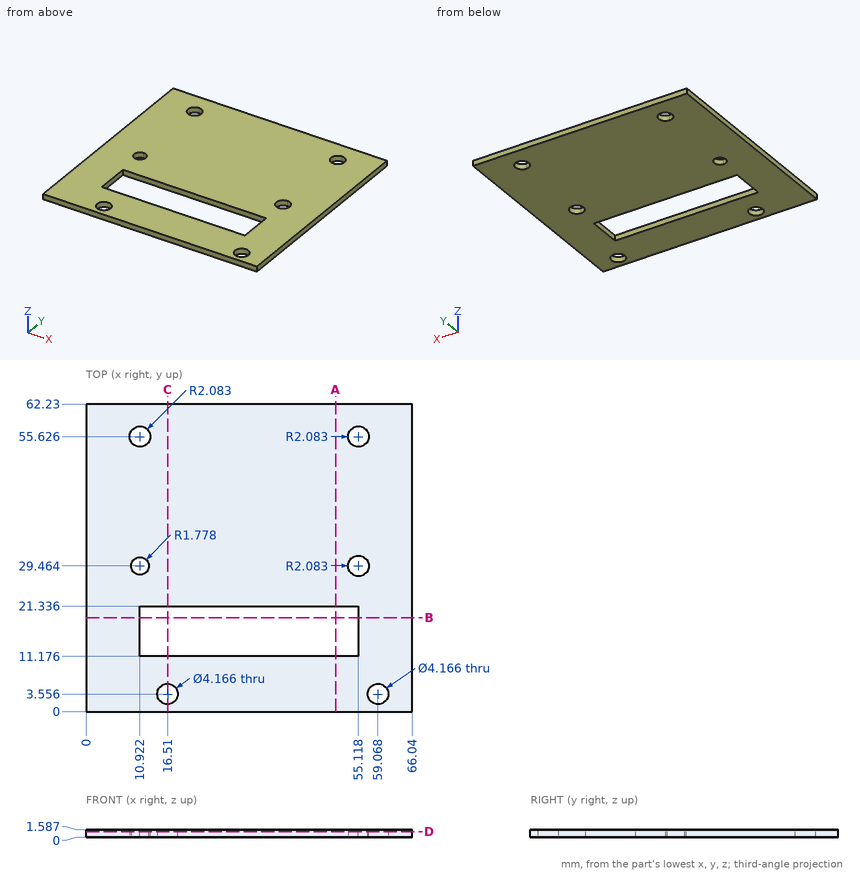
Geometry: see drawing. Coordinates: mm, zero at the bounding-box minimum. Coordinates: 2 decimals unless noted, no trailing zeros. Loops run counter-clockwise (first coordinate to the right, second up) from the corner with the lowest first, then second, coordinate; pieces in that order, holes last. Notation, with made-up numbers: (-12, 77) - (43, 77) arc R20 ccw to (43, 108) - close; hole circle Ø10 at (72.25, 21.25). An arc over 180 degrees is marked (long way). Put each result on its own line as item: value. Start each with the question number.
Q1. Cut plane A-A, the plane x = 50.5. Return loops of the section in (y, z) (1 decimal).
Q2. Cut plane D-D, the plane z = 1.15. Return loops of the section in (x, y) (1 decimal), and give its area (3 significant figures).
Q3. Line query: line 1 (Y direction, x = 16.51, z = 0.4) (1 decimal); line 2 (Y direction, x = 42.5, z = 1.15) (1 decimal); line 3 (X direction, y = 18.5, z = 1.5). Output: solid intervals per line, ascending.
Q4. Cut plane B-B, the plane y = 19. Return loops of the section in (x, z).
Q5. Cut plane C-C, the plane x = 16.51. Return loops of the section in (y, z) (1 decimal).
Filled sheet:
1. outline: (0, 0) - (11.2, 0) - (11.2, 1.6) - (0, 1.6) - close; (21.3, 0) - (62.2, 0) - (62.2, 1.6) - (21.3, 1.6) - close
2. outline: (0, 0) - (66, 0) - (66, 62.2) - (0, 62.2) - close; hole circle Ø4.2 at (10.9, 55.6); hole circle Ø3.6 at (10.9, 29.5); hole (10.9, 11.2) - (55.1, 11.2) - (55.1, 21.3) - (10.9, 21.3) - close; hole circle Ø4.2 at (16.5, 3.6); hole circle Ø4.2 at (55.1, 29.5); hole circle Ø4.2 at (55.1, 55.6); hole circle Ø4.2 at (59.1, 3.6)
2. area: 3,580 mm²
3. line 1: 0 to 1.5, 5.6 to 11.2, 21.3 to 62.2
3. line 2: 0 to 11.2, 21.3 to 62.2
3. line 3: 0 to 10.92, 55.12 to 66.04
4. outline: (0, 0) - (10.92, 0) - (10.92, 1.59) - (0, 1.59) - close; (55.12, 0) - (66.04, 0) - (66.04, 1.59) - (55.12, 1.59) - close
5. outline: (0, 0) - (1.5, 0) - (1.5, 1.6) - (0, 1.6) - close; (5.6, 0) - (11.2, 0) - (11.2, 1.6) - (5.6, 1.6) - close; (21.3, 0) - (62.2, 0) - (62.2, 1.6) - (21.3, 1.6) - close
